Work out the finished part from the listing and answer in its coordinate system (mm). A direction names the side the tool comes from. Round coordinates to 2 decimals unless told otherwise and drop trailing zeros. Write each loop counter-clockwise with the first axis right and the second up, starting at its lowest first coordinate (ties: lowest second). Pieces come first, ordered by that corner, then holes.
from build123d import *

# Parameters (mm, degrees)
SKETCH1_R           = 13.843
BOSS_EXTRUDE1_DEPTH = 46.482
SKETCH2_R           = 4.9657
BOSS_EXTRUDE2_DEPTH = 3.3528
SKETCH3_R           = 4.953
BOSS_EXTRUDE3_DEPTH = 2.8956
BOSS_EXTRUDE4_DEPTH = 9.2583
SKETCH5_R           = 1.11125
SKETCH5_R_2         = 1.21285
CUT_EXTRUDE1_DEPTH  = 5.4356
MIRROR1_START       = 41.0464
MIRROR1_DEPTH       = 5.4356


# Read off the part's stored shape, not the designer's step: Mirror1
with BuildPart() as part:
    # Sketch1 → Boss-Extrude1 (new body)
    with BuildSketch(Plane(origin=(0, 0, 0), x_dir=(1, 0, 0), z_dir=(0, 1, 0))):
        with Locations(Location((0, 0, 0), (0, 0, 270))):
            Circle(SKETCH1_R)
    extrude(amount=BOSS_EXTRUDE1_DEPTH)

    # Sketch2 → Boss-Extrude2 (add)
    with BuildSketch(Plane(origin=(0, 46.482, 0), x_dir=(1, 0, 0), z_dir=(0, 1, 0))):
        with Locations(Location((0, 0, 0), (0, 0, 270))):
            Circle(SKETCH2_R)
    extrude(amount=BOSS_EXTRUDE2_DEPTH)

    # Sketch3 → Boss-Extrude3 (add)
    with BuildSketch(Plane.XZ):
        with Locations(Location((0, 0, 0), (0, 0, 270))):
            Circle(SKETCH3_R)
    extrude(amount=BOSS_EXTRUDE3_DEPTH)

    # Sketch4 → Boss-Extrude4 (add)
    with BuildSketch(Plane(origin=(0, 49.8348, 0), x_dir=(1, 0, 0), z_dir=(0, 1, 0))):
        with BuildLine():
            Line((-1.047576804, -0.4572), (1.047576804, -0.4572))
            ThreePointArc((1.047576804, -0.4572), (0, 1.143), (-1.047576804, -0.4572))
        make_face()
    extrude(amount=BOSS_EXTRUDE4_DEPTH)

    # Sketch5 → Cut-Extrude1 (cut)
    with BuildSketch(Plane(origin=(0, 46.482, 0), x_dir=(1, 0, 0), z_dir=(0, 1, 0))):
        with Locations(Location((0, 7.70255, 0), (0, 0, 270))):
            Circle(SKETCH5_R)
        with Locations(Location((0, -7.70255, 0), (0, 0, 270))):
            Circle(SKETCH5_R)
        with Locations(Location((-10.29335, 0, 0), (0, 0, 270))):
            Circle(SKETCH5_R_2)
        with BuildLine():
            ThreePointArc((-5.018539731, 5.564108911), (-5.941000388, 4.566132214), (-6.668031862, 3.417952617))
            ThreePointArc((-6.668031862, 3.417952617), (-8.668133869, 2.773445377), (-9.312641109, 4.773547383))
            ThreePointArc((-9.312641109, 4.773547383), (-8.297261558, 6.377106685), (-7.008943624, 7.770891089))
            ThreePointArc((-7.008943624, 7.770891089), (-4.910350588, 7.662701947), (-5.018539731, 5.564108911))
        make_face()
        with BuildLine():
            ThreePointArc((-6.668031862, -3.417952617), (-8.668133869, -2.773445377), (-9.312641109, -4.773547383))
            ThreePointArc((-9.312641109, -4.773547383), (-8.297261558, -6.377106685), (-7.008943624, -7.770891089))
            ThreePointArc((-7.008943624, -7.770891089), (-4.910350588, -7.662701947), (-5.018539731, -5.564108911))
            ThreePointArc((-5.018539731, -5.564108911), (-5.941000388, -4.566132214), (-6.668031862, -3.417952617))
        make_face()
    extrude(amount=-CUT_EXTRUDE1_DEPTH, mode=Mode.SUBTRACT)

    # Mirror1 outline → Mirror1 (cut)
    with BuildSketch(Plane(origin=(0, 0, 0), x_dir=(1, 0, 0), z_dir=(0, 1, 0)).offset(MIRROR1_START)):
        with BuildLine():
            ThreePointArc((7.008943624, -7.770891089), (8.297261558, -6.377106685), (9.312641109, -4.773547383))
            ThreePointArc((9.312641109, -4.773547383), (8.668133868, -2.773445377), (6.668031862, -3.417952617))
            ThreePointArc((6.668031862, -3.417952617), (5.941000388, -4.566132214), (5.018539731, -5.564108911))
            ThreePointArc((5.018539731, -5.564108911), (4.910350588, -7.662701947), (7.008943624, -7.770891089))
        make_face()
        with BuildLine():
            ThreePointArc((6.668031862, 3.417952617), (8.668133868, 2.773445377), (9.312641109, 4.773547383))
            ThreePointArc((9.312641109, 4.773547383), (8.297261558, 6.377106685), (7.008943624, 7.770891089))
            ThreePointArc((7.008943624, 7.770891089), (4.910350588, 7.662701947), (5.018539731, 5.564108911))
            ThreePointArc((5.018539731, 5.564108911), (5.941000388, 4.566132214), (6.668031862, 3.417952617))
        make_face()
    extrude(amount=MIRROR1_DEPTH, mode=Mode.SUBTRACT)


solid = part.part
Q1. Find section A-A (x = 0). Determine the outline of the cut face in (y, z).
Q2. Find section C-C (z = 9.5). Determine the outline of the cut face in (x, y).
Q3. A tool of negligible diameter and unlimited length cuts with its end or side. For faces 1 (the face through (11.7, 22.9, 7.4)), 2 (the face through (1.488, -1.428, -4.724)), 3 (the face through (0, 54, 0.457)), 4 (the face through (-5.93, 43.8, -4.58)), from which of +Z, -Z, +X, -X, +Y, -Y can it reach the whole face along a straight path? Write none if from no direction.
Q4. Given pin 1 (2 mm diameter, centred on x = -10, y = 23.5, fed in from +Z); pin 2 (3 mm diameter, centred on x = 0, z = 7.7, fed in from -Y); pin 3 (4 mm diameter, centred on x = 8.5, y = 26, fed in from +Z), each flat-ended and moving along its own axis, determine where each tip first touches the part or whether it passes through.
Q5. Find section B-B (y = 4.5). Determine the outline of the cut face in (x, z).
Q6. Find the intervals of material crossed by L1, parallel to Y at x = -3.5, z = 0.75; L2, parallel to Y at x = 5.75, z = -2.25; L3, parallel to Z at x = 9, y = 42, in increasing order.
Q7. Find section D-D (x = -5.75). Determine the outline of the cut face in (y, z), plus the area to 3 significant figures.
Report:
1. outline: (-2.9, -4.95) - (0, -4.95) - (0, -13.84) - (46.48, -13.84) - (46.48, -8.81) - (41.05, -8.81) - (41.05, -6.59) - (46.48, -6.59) - (46.48, -4.97) - (49.83, -4.97) - (49.83, -1.14) - (59.09, -1.14) - (59.09, 0.46) - (49.83, 0.46) - (49.83, 4.97) - (46.48, 4.97) - (46.48, 6.59) - (41.05, 6.59) - (41.05, 8.81) - (46.48, 8.81) - (46.48, 13.84) - (0, 13.84) - (0, 4.95) - (-2.9, 4.95) - close
2. outline: (-10.07, 0) - (10.07, 0) - (10.07, 46.48) - (-10.07, 46.48) - close
3. face 1: +Y, -Y
3. face 2: -Y
3. face 3: +Z, +X, -X, +Y
3. face 4: +Y
4. pin 1: stops at z = 10.52
4. pin 2: stops at y = 0
4. pin 3: stops at z = 12.22
5. outline: circle Ø27.69 at (0, 0)
6. L1: y = -2.9 to 49.83
6. L2: y = 0 to 46.48
6. L3: z = -10.52 to -5.34, -3.01 to 3.01, 5.34 to 10.52
7. outline: (0, -12.59) - (46.48, -12.59) - (46.48, -8.13) - (41.05, -8.13) - (41.05, -4.8) - (46.48, -4.8) - (46.48, 4.8) - (41.05, 4.8) - (41.05, 8.13) - (46.48, 8.13) - (46.48, 12.59) - (0, 12.59) - close
7. area: 1,130 mm2
